Verification items for this drawing (mm, ordinates from the low corner). Round coordinates to 2 decimals unless told otherwise and drop trailing zeros. Order: outer loops, then holes, each group sorted by start corner. A loop starts at its lowest first (then second) coordinate and runs counter-clockwise, first axis right, second up. Notation, with made-up numbers: (-10.75, 48.5) - (7.25, 48.5) arc R26 cw to (7.25, 68.5) - close; hole circle Ø4 at (86.25, -12.5). An arc over 180 degrees is marked (long way). Answer as CSV lines item,"result". Start each with the question number.
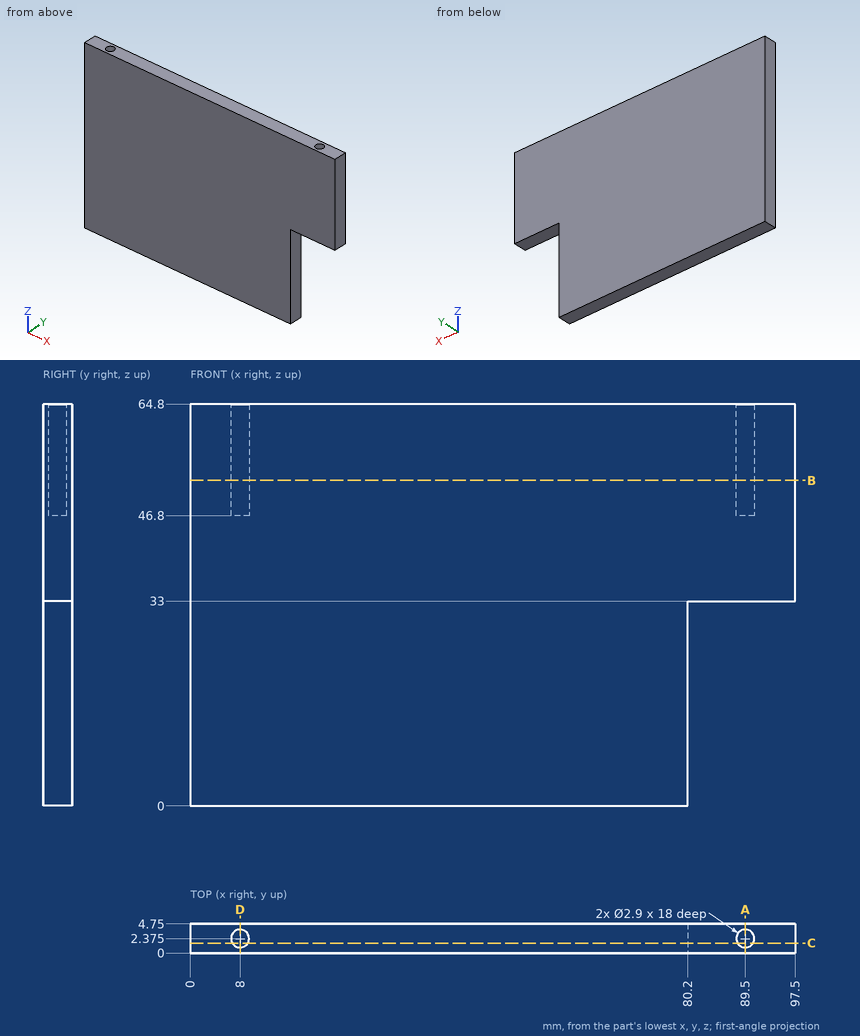
1. Section check C-C on y = 1.65. Record the boundary of the cut face in (x, z), plus the area to 3 significant figures.
2. Section check D-D on x = 8. Record the boundary of the cut face in (y, z) (3 decimals).
3. Go/stop test with flat-tipped pins: pin 1 Ø1.7 at (x, y) = (89.5, 2.375) entering from -Z; pin 2 Ø1.5 at (x, y) = (89.5, 2) entering from +Z; pin 3 Ø2.5 at (x, y) = (8, 1.5) entering from +Z. Record where each tip stops, or that it passes through.
4. Section check A-A on x = 89.5. Record the boundary of the cut face in (y, z) (3 decimals).
5. Section check B-B on z = 52.5. Record the boundary of the cut face in (x, y) (3 decimals).
6. Thickness scan on probe 1 along Y at (x, z) = (89.5, 51.5) (3 decimals); probe 2 along X at (y, z) = (1.3, 47); probe 3 along X at (y, z) = (1.15, 59.5). Record the ranges inside material, lowest first.
Numbers:
1,outline,"(0, 0) - (80.2, 0) - (80.2, 33) - (97.5, 33) - (97.5, 64.8) - (90.76, 64.8) - (90.76, 46.8) - (88.24, 46.8) - (88.24, 64.8) - (9.26, 64.8) - (9.26, 46.8) - (6.74, 46.8) - (6.74, 64.8) - (0, 64.8) - close"
1,area,"5,660 mm2"
2,outline,"(0, 0) - (4.75, 0) - (4.75, 64.8) - (3.825, 64.8) - (3.825, 46.8) - (0.925, 46.8) - (0.925, 64.8) - (0, 64.8) - close"
3,pin 1,"stops at z = 33"
3,pin 2,"stops at z = 46.8"
3,pin 3,"stops at z = 64.8"
4,outline,"(0, 33) - (4.75, 33) - (4.75, 64.8) - (3.825, 64.8) - (3.825, 46.8) - (0.925, 46.8) - (0.925, 64.8) - (0, 64.8) - close"
5,outline,"(0, 0) - (97.5, 0) - (97.5, 4.75) - (0, 4.75) - close; hole circle Ø2.9 at (8, 2.375); hole circle Ø2.9 at (89.5, 2.375)"
6,probe 1,"y = 0 to 0.925, 3.825 to 4.75"
6,probe 2,"x = 0 to 7.03, 8.97 to 88.53, 90.47 to 97.5"
6,probe 3,"x = 0 to 7.22, 8.78 to 88.72, 90.28 to 97.5"
